Part model, mm, in its own coordinate system. Round coordinates to 2 decimals unless told otherwise and drop trailing zeros. Order: outer loops, then holes, each group sorted by start corner. A loop starts at its lowest first (then second) coordinate and runs counter-clockwise, first axis right, second up. Notation, with made-up numbers: (81, -37) - (128, -37) arc R10 cw to (128, -19) - close; hole circle Ø1 at (-24.75, 67.25). An arc over 180 degrees is marked (long way). Answer as a JSON object with one key per item and string values.
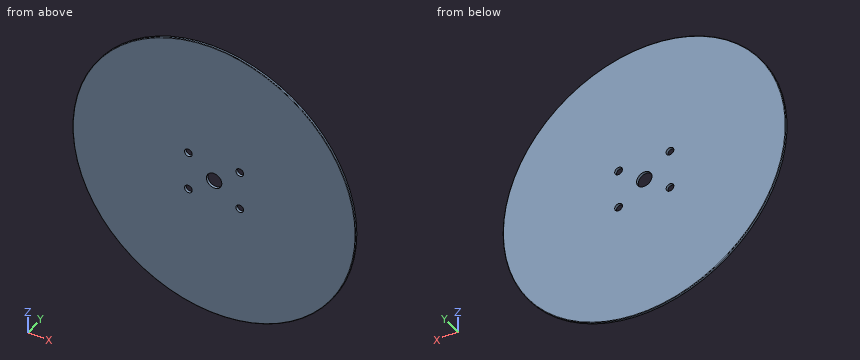
```python
from build123d import *

# Parameters (mm, degrees)
SKETCH1_R           = 55
BOSS_EXTRUDE1_DEPTH = 1
FILLET2_R           = 0.2
SKETCH4_R           = 3
CUT_EXTRUDE2_DEPTH  = 2
SKETCH3_R           = 1.5
CUT_EXTRUDE3_DEPTH  = 2


with BuildPart() as part:
    # Sketch1 → Boss-Extrude1 (new body)
    with BuildSketch(Plane(origin=(0, 0, 0), x_dir=(1, 0, 0), z_dir=(0, 1, 0))):
        Circle(SKETCH1_R)
    extrude(amount=BOSS_EXTRUDE1_DEPTH)

    # Fillet2
    fillet2_edges = [part.edges().sort_by_distance(p)[0] for p in [
        (-55, 0, 0),
        (-55, 1, 0),
    ]]
    fillet(fillet2_edges, radius=FILLET2_R)

    # Sketch4 → Cut-Extrude2 (cut, through all)
    with BuildSketch(Plane(origin=(0, 1, 0), x_dir=(1, 0, 0), z_dir=(0, 1, 0))):
        Circle(SKETCH4_R)
    extrude(amount=-CUT_EXTRUDE2_DEPTH, mode=Mode.SUBTRACT)

    # Sketch3 → Cut-Extrude3 (cut, through all)
    with BuildSketch(Plane(origin=(0, 1, 0), x_dir=(1, 0, 0), z_dir=(0, 1, 0))):
        with Locations((-10, 7.5)):
            Circle(SKETCH3_R)
        with Locations((10, 7.5)):
            Circle(SKETCH3_R)
        with Locations((10, -7.5)):
            Circle(SKETCH3_R)
        with Locations((-10, -7.5)):
            Circle(SKETCH3_R)
    extrude(amount=-CUT_EXTRUDE3_DEPTH, mode=Mode.SUBTRACT)


solid = part.part
```
Item 1: Cut at C-C (y = 0.6). Write the cut outline in (x, z).
Taken from the geometry:
{"outline": "circle Ø110 at (0, 0); hole circle Ø3 at (-10, -7.5); hole circle Ø3 at (-10, 7.5); hole circle Ø6 at (0, 0); hole circle Ø3 at (10, -7.5); hole circle Ø3 at (10, 7.5)"}
Item 2: Cut at A-A (x = 0). Write the cut outline in (y, z), plus the area to 3 significant figures.
Taken from the geometry:
{"outline": "(0, -54.8) arc R0.2 ccw to (0.2, -55) - (0.8, -55) arc R0.2 ccw to (1, -54.8) - (1, -3) - (0, -3) - close; (0, 3) - (1, 3) - (1, 54.8) arc R0.2 ccw to (0.8, 55) - (0.2, 55) arc R0.2 ccw to (0, 54.8) - close", "area": "104 mm2"}
Item 3: Cut at B-B (z = 0). Write the cut outline in (x, y).
Taken from the geometry:
{"outline": "(-55, 0.2) arc R0.2 ccw to (-54.8, 0) - (-3, 0) - (-3, 1) - (-54.8, 1) arc R0.2 ccw to (-55, 0.8) - close; (3, 0) - (54.8, 0) arc R0.2 ccw to (55, 0.2) - (55, 0.8) arc R0.2 ccw to (54.8, 1) - (3, 1) - close"}
Item 4: Drop a flat-ended pin along its axis: P1, Ø2.5, axis at x = 10, z = -7.5, coming from the -Y side. Give the stop position or say it passes through.
Taken from the geometry:
{"P1": "through"}
Item 5: Probe L1, parallel to Z at x = 10, y = 0.55; L2, parallel to X at y = 0.75, z = 7.5; L3, parallel to X at y = 0.6, z = 7. List the from-to ranges inside material, lowest first. Write a range as from..to.
Taken from the geometry:
{"L1": "-54.08..-9, -6..6, 9..54.08", "L2": "-54.49..-11.5, -8.5..8.5, 11.5..54.49", "L3": "-54.55..-11.41, -8.59..8.59, 11.41..54.55"}
